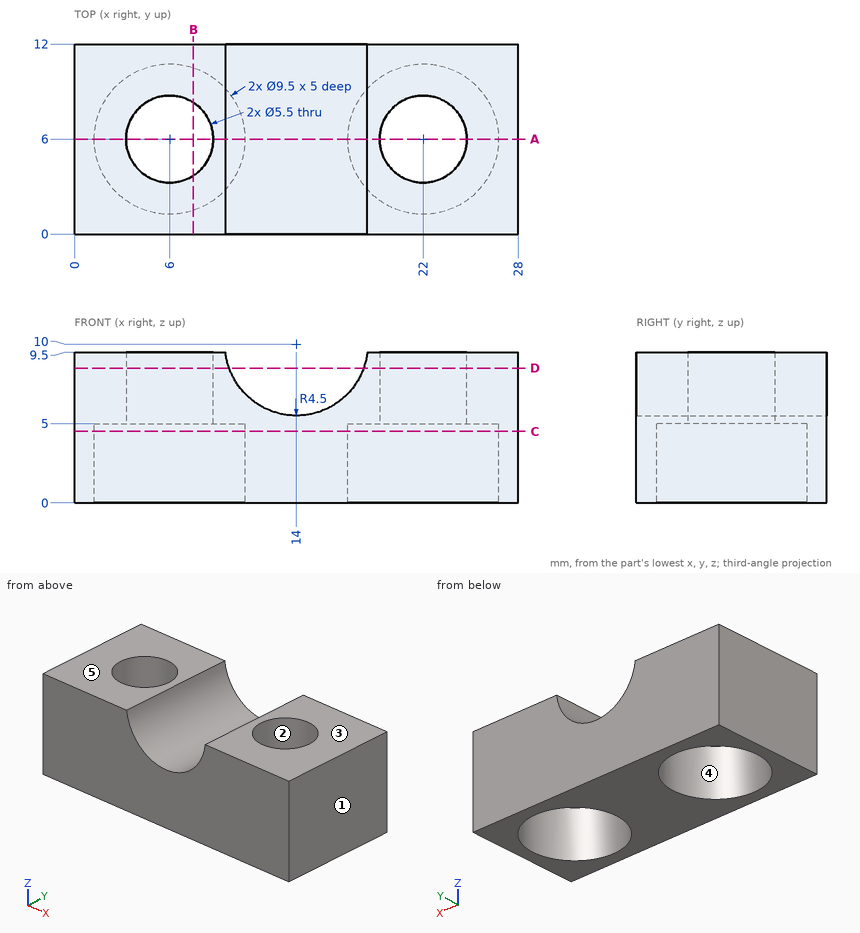
Here's the drawing with two shaded views (mm, measured from the low corner). I have some questions. A direction names the side the tool comes from. Coordinates: 2 decimals unless noted, no trailing zeros. Write each loop counter-clockwise with the first axis right and the second up, starting at its lowest first coordinate (ties: lowest second). Pieces come first, ordered by that corner, then holes. Notation, with made-up numbers: (10, -5) -> (52, -5) arc R29 cw to (52, 19) -> close; hole circle Ø2 at (15, 7.5). An arc over 180 degrees is marked (long way). Write item = value, one per line. Start each with the question number.
(1) Which directions (+Z, -Z, +X, -X, +Y, -Y) give clear straight access to the entire face, cutting with the end or side of a thin tool? Please do the marked faces 4 and 5.
(2) I want a section at B-B (x = 7.5). Please give me the cut outline in (y, z).
(3) I want a section at D-D (z = 8.5). Please give me the cut outline in (x, y), plus the area to 3 significant figures.
(4) I want a section at A-A (y = 6). Please give me the cut outline in (x, z).
(5) We'd pull the mould along X, two halves only. Please class the marked faces 1, 2 and 3: released by +X, released by -X, zero draft, split by the parting line, or undercut.
(6) Will these pins go through, and if not, where does the flat tip stop? pin 1 (2 mm diameter, centred on x = 17, y = 2.5, fed in from +Z); pin 2 (3 mm diameter, centred on x = 20.5, y = 8.5, fed in from -Z).
(7) I want a section at C-C (z = 4.5). Please give me the cut outline in (x, y).
(8) I need wall thicknesses on line 1 (Y direction, x = 6, z = 6.9); line 2 (X direction, y = 7, z = 0.75); line 3 (X direction, y = 6, z = 6.9). Which ranges of each line are inside material? Lowest first, please. Write a range as [from, to].
Result set:
q1.face_4 = -Z
q1.face_5 = +Z, +X, -X, +Y, -Y
q2.outline = (0, 0) -> (1.49, 0) -> (1.49, 5) -> (3.7, 5) -> (3.7, 9.5) -> (0, 9.5) -> close; (8.3, 5) -> (10.51, 5) -> (10.51, 0) -> (12, 0) -> (12, 9.5) -> (8.3, 9.5) -> close
q3.outline = (0, 0) -> (9.76, 0) -> (9.76, 12) -> (0, 12) -> close; (18.24, 0) -> (28, 0) -> (28, 12) -> (18.24, 12) -> close; hole circle Ø5.5 at (6, 6); hole circle Ø5.5 at (22, 6)
q3.area = 187 mm2
q4.outline = (0, 0) -> (1.25, 0) -> (1.25, 5) -> (3.25, 5) -> (3.25, 9.5) -> (0, 9.5) -> close; (8.75, 5) -> (10.75, 5) -> (10.75, 0) -> (17.25, 0) -> (17.25, 5) -> (19.25, 5) -> (19.25, 9.5) -> (18.47, 9.5) arc R4.5 cw to (9.53, 9.5) -> (8.75, 9.5) -> close; (24.75, 5) -> (26.75, 5) -> (26.75, 0) -> (28, 0) -> (28, 9.5) -> (24.75, 9.5) -> close
q5.face_1 = released by +X
q5.face_2 = undercut
q5.face_3 = zero draft
q6.pin_1 = 7.94
q6.pin_2 = 5
q7.outline = (0, 0) -> (28, 0) -> (28, 12) -> (0, 12) -> close; hole circle Ø9.5 at (6, 6); hole circle Ø9.5 at (22, 6)
q8.line_1 = [0, 3.25], [8.75, 12]
q8.line_2 = [0, 1.36], [10.64, 17.36], [26.64, 28]
q8.line_3 = [0, 3.25], [8.75, 10.74], [17.26, 19.25], [24.75, 28]
